Study the drawing (mm; zero at the part's minimum x, y, z) and answer. A direction names the side the tool comes from. Round coordinates to 2 decimals unless told otherwise and drop trailing zeros. Order: outer loops, then holes, each group sorted by start corner. A loop starts at its lowest first (then second) coordinate and runs counter-clockwise, first axis right, second up. Notation, with made-up numbers: (87, -5.5) -> (130, -5.5) arc R9 cw to (130, 0.5) -> close; hole circle Ø6 at (70.5, 27.25). An arc over 180 degrees is marked (long way). Answer in a Markdown table with one row per item. Add a question column.
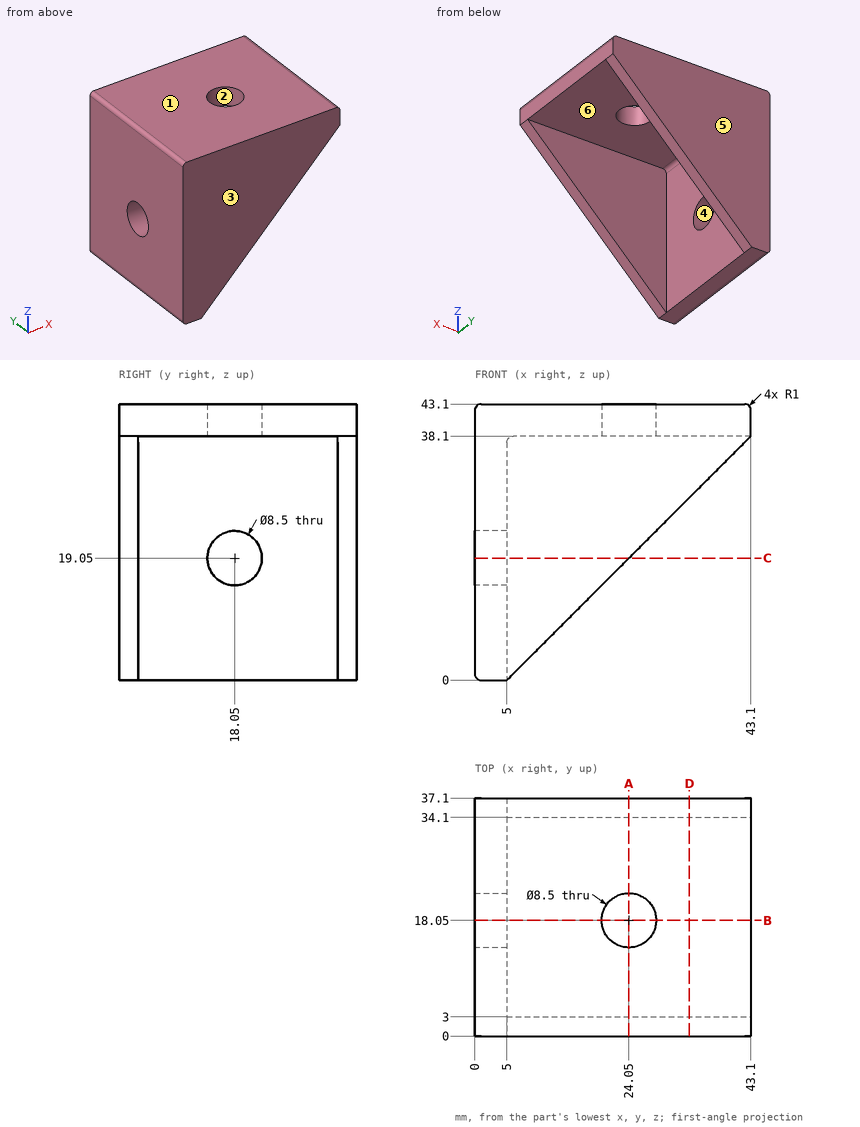
Item 1: For a pull along Y with two mould halves and no side action, classify the marked faces 1, 2, 3 and 4 as released by +Y, released by -Y, zero draft, split by the parting line, or undercut.
Item 2: Find the intervals of material crossed by probe 1 along X at (y, z) = (18, 39); probe 2 along Y at (x, z) = (24.05, 41.7); probe 3 along Y at (x, z) = (27, 35), in increasing order. Write a range as [from, to].
Item 3: A tool of negligible diameter and unlimited length cuts with its end or side. For the marked faces 5 and 6, from which of +Z, -Z, +X, -X, +Y, -Y can it reach the whole face along a straight path? Write none if from no direction.
Item 4: The part is cut by section D-D, the plane x = 33.5. Give the vertices of the cut face in (y, z).
Item 5: The part is cut by section A-A, the plane x = 24.05. Give the vertices of the cut face in (y, z).
Item 6: The part is cut by section B-B, the plane y = 18.05. Give the vertices of the cut face in (x, z), and give its area (3 significant figures).
Item 7: The part is cut by section C-C, the plane z = 19.05. Give the vertices of the cut face in (x, y).
Item 8: Flat-ended cylindrical pins translate along their axes: P1, Ø9.5, axis at y = 20, z = 24, coming from the +X side; P2, Ø5, axis at x = 32, y = 18, coming from the -Z side. Find the tip coordinate at first contact, or state that the pin passes through.
Resolved:
| question | item | result |
|---|---|---|
| 1 | face 1 | zero draft |
| 1 | face 2 | undercut |
| 1 | face 3 | released by -Y |
| 1 | face 4 | undercut |
| 2 | probe 1 | [0, 19.8], [28.3, 43.1] |
| 2 | probe 2 | [0, 13.8], [22.3, 37.1] |
| 2 | probe 3 | [0, 3], [34.1, 37.1] |
| 3 | face 5 | +Z, -Z, +X, -X, +Y |
| 3 | face 6 | -Z, +X |
| 4 | outline | (0, 28.5) -> (3, 28.5) -> (3, 38.1) -> (34.1, 38.1) -> (34.1, 28.5) -> (37.1, 28.5) -> (37.1, 43.1) -> (0, 43.1) -> close |
| 5 | outline | (0, 19.05) -> (3, 19.05) -> (3, 38.1) -> (13.8, 38.1) -> (13.8, 43.1) -> (0, 43.1) -> close; (22.3, 38.1) -> (34.1, 38.1) -> (34.1, 19.05) -> (37.1, 19.05) -> (37.1, 43.1) -> (22.3, 43.1) -> close |
| 6 | outline | (0, 1) arc R1 ccw to (1, 0) -> (5, 0) -> (5, 14.8) -> (0, 14.8) -> close; (0, 23.3) -> (5, 23.3) -> (5, 37.1) arc R1 cw to (6, 38.1) -> (19.8, 38.1) -> (19.8, 43.1) -> (1, 43.1) arc R1 ccw to (0, 42.1) -> close; (28.3, 38.1) -> (43.1, 38.1) -> (43.1, 42.1) arc R1 ccw to (42.1, 43.1) -> (28.3, 43.1) -> close |
| 6 | area | 321 mm2 |
| 7 | outline | (0, 0) -> (24.05, 0) -> (24.05, 3) -> (5, 3) -> (5, 13.8) -> (0, 13.8) -> close; (0, 22.3) -> (5, 22.3) -> (5, 34.1) -> (24.05, 34.1) -> (24.05, 37.1) -> (0, 37.1) -> close |
| 8 | P1 | x = 5 |
| 8 | P2 | z = 38.1 |
